Study the drawing (mm; zero at the part's minimum x, y, z) and answer. A direction names the side the tool comes from. Round coordinates to 2 decimals unless told otherwise and drop trailing zeros. Loops run counter-clockwise (first coordinate to the right, second up) from the corner with the lowest first, then second, coordinate; pieces in that order, holes last. Notation, with made-up numbers: (-18.5, -3) -> (29.5, -3) arc R14 cw to (29.5, 12) -> close; hole circle Ø9 at (-21, 18.5). An arc over 180 degrees is marked (long way). Write each question's results on one line, items separated by ' | '. Start each with the question number.
(1) For the marked faces 4 and 5, determine the directions among +Z, -Z, +X, -X, +Y, -Y from which every point of the face is accessible in a straight line to the end or side of a thin tool.
(2) The part is cut by section D-D (x = 4.1). Determine the outline of the cut face in (y, z).
(3) The part is cut by section B-B (y = 4.25). Determine the outline of the cut face in (x, z).
(4) The part is cut by section A-A (z = 2.25). Determine the outline of the cut face in (x, y) (1 decimal).
(5) Flat-ended cylindrical pins translate along their axes: pin 1 (2 mm diameter, centred on x = 1, z = 8, fed in from -Y); pin 2 (3 mm diameter, centred on x = 2.98, y = 3.45, fed in from +Z). Find the tip coordinate at first contact, or state that the pin passes through.
(6) Straight lines are drawn through the part: probe 1 along X at (y, z) = (3, 10.25); probe 2 along Y at (x, z) = (3.1, 2.5) (1 decimal); probe 3 along Y at (x, z) = (1.9, 4.25) (1 decimal). For each, find the intervals that lie inside material, in ascending order.
(7) Determine the mould class of the marked faces 1, 2 and 3 for opening direction Y: released by +Y, released by -Y, zero draft, split by the parting line, or undercut.
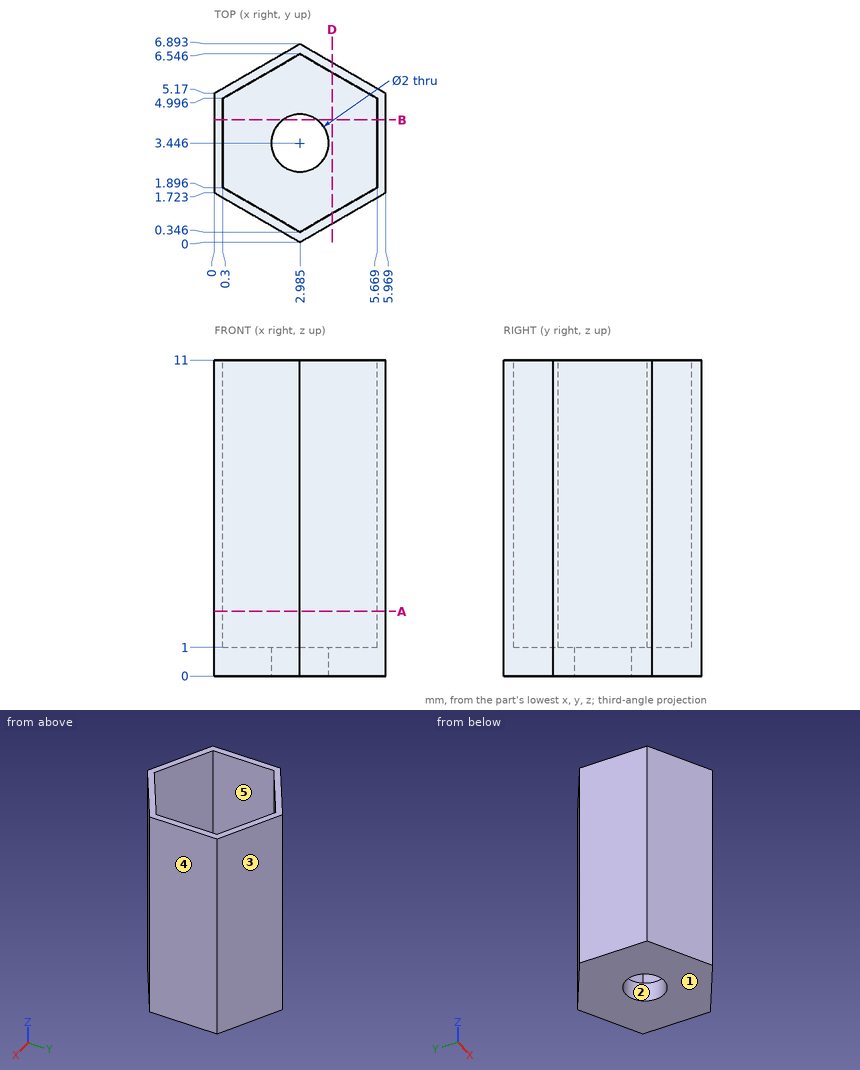
Checked values:
1) face 4: +Z, -Z, +X, +Y, -Y | face 5: +Z
2) outline: (0.64, 0) -> (6.25, 0) -> (6.25, 11) -> (5.9, 11) -> (5.9, 1) -> (0.99, 1) -> (0.99, 11) -> (0.64, 11) -> close
3) outline: (0, 0) -> (2.39, 0) -> (2.39, 1) -> (0.3, 1) -> (0.3, 11) -> (0, 11) -> close; (3.58, 0) -> (5.97, 0) -> (5.97, 11) -> (5.67, 11) -> (5.67, 1) -> (3.58, 1) -> close
4) outline: (0, 1.7) -> (3, 0) -> (6, 1.7) -> (6, 5.2) -> (3, 6.9) -> (0, 5.2) -> close; hole (0.3, 1.9) -> (3, 0.3) -> (5.7, 1.9) -> (5.7, 5) -> (3, 6.5) -> (0.3, 5) -> close
5) pin 1: stops at y = 0.57 | pin 2: stops at z = 1
6) probe 1: x = 0 to 0.3, 5.67 to 5.97 | probe 2: y = 0.1 to 0.4, 6.5 to 6.8 | probe 3: y = 0.6 to 1, 5.9 to 6.3
7) face 1: zero draft | face 2: undercut | face 3: released by +Y
